Print and shaded views of the part. All mm, measured from the part's lowest x, y and z. A direction names the side the tool comes from. Round coordinates to 2 decimals unless told otherwise and drop trailing zeros. Order: outer loops, then holes, each group sorted by start corner. A loop starts at its lowest first (then second) coordinate and runs counter-clockwise, first axis right, second up. Notation, with made-up numbers: (85.5, 3.25) - (109.5, 3.25) arc R5 cw to (109.5, 10.25) - close; hole circle Ø2 at (-16, -25.75). An arc over 180 degrees is marked (long way). Return JSON: item names as keys, results as strings. Group by question number.
Item 1: Saw through at C-C on x = 10. List the corners of the cut face in (y, z).
Item 2: Saw through at B-B on z = 10.5. List the corners of the cut face in (x, y).
Item 3: Saw through at D-D on z = 18.5. List the corners of the cut face in (x, y), and give its area (3 significant figures).
Item 4: Tool access for the marked faces 5, 6, 7 and 8: list every direction of +Z, -Z, +X, -X, +Y, -Y with a clear straight run to the whole face (end or side of a thin tool).
Item 5: Saw through at A-A on y = 8.5. List the corners of the cut face in (x, z).
Item 6: Drop flat-ended pins along their axis: pin 1 (25 mm diameter, centred on x = 53, z = 34.5, fed in from -Y); pin 2 (11.5 mm diameter, centred on x = 108, z = 60, fed in from +Y); pin 3 (1.5 mm diameter, centred on y = 11.5, z = 52.5, fed in from +X). Give the stop position or say it passes through.
Item 7: Probe probe 1 along Y at (x, z) = (46, 16); probe 2 along Z at (x, y) = (112, 8) (1 decimal); probe 3 along Y at (x, z) = (103, 28.5). List the from-to ranges inside material, lowest first.
Item 8: Two-plate mould, pull along Z, no slides. Class the marked faces 1, 2, 3 and 4: released by +Z, released by -Z, zero draft, split by the parting line, or undercut.
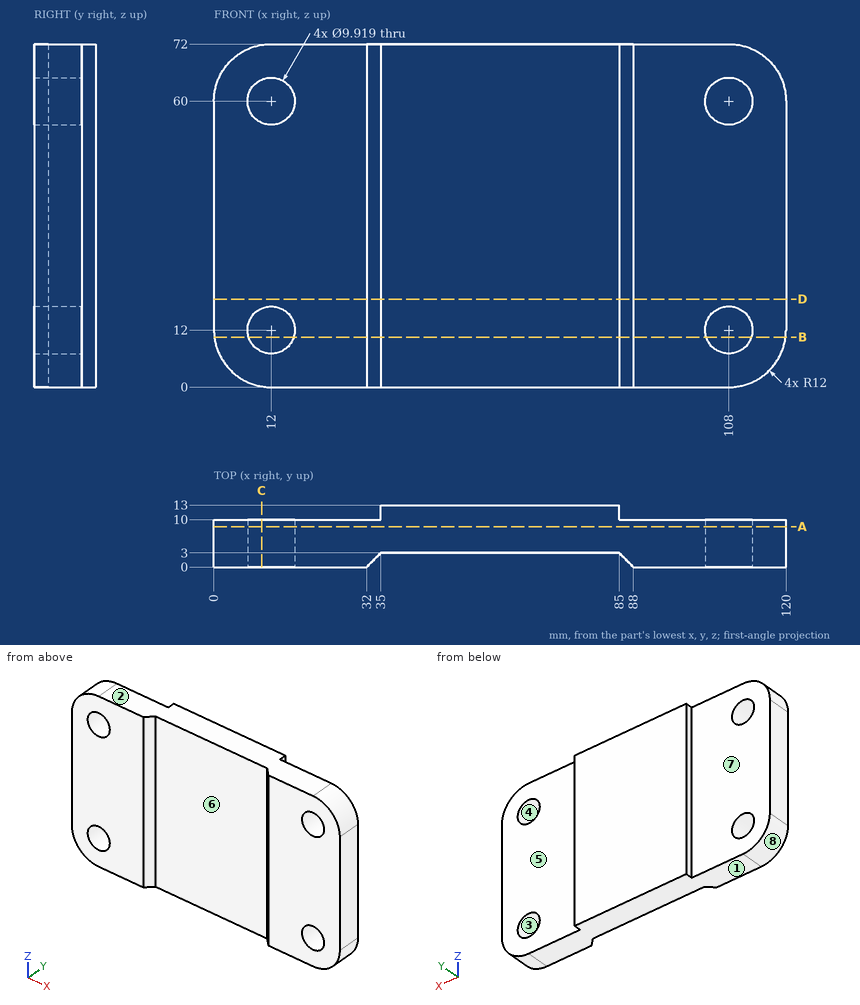
Filled in:
{
 "1": {"outline": "(0, 0.17) - (10, 0.17) - (10, 7.46) - (0, 7.46) - close; (0, 16.54) - (10, 16.54) - (10, 55.46) - (0, 55.46) - close; (0, 64.54) - (10, 64.54) - (10, 71.83) - (0, 71.83) - close"},
 "2": {"outline": "(0.09, 0) - (7.27, 0) - (7.27, 10) - (0.09, 10) - close; (16.73, 0) - (32, 0) - (35, 3) - (85, 3) - (88, 0) - (103.27, 0) - (103.27, 10) - (85, 10) - (85, 13) - (35, 13) - (35, 10) - (16.73, 10) - close; (112.73, 0) - (119.91, 0) - (119.91, 10) - (112.73, 10) - close"},
 "3": {"outline": "(0, 0) - (32, 0) - (35, 3) - (85, 3) - (88, 0) - (120, 0) - (120, 10) - (85, 10) - (85, 13) - (35, 13) - (35, 10) - (0, 10) - close", "area": "1,190 mm^2"},
 "4": {"face 5": "+Z, -Z, +X, +Y", "face 6": "+Z, -Z, -Y", "face 7": "+Z, -Z, -X, +Y", "face 8": "-Z, -X, +Y, -Y"},
 "5": {"outline": "(0, 12) arc R12 ccw to (12, 0) - (108, 0) arc R12 ccw to (120, 12) - (120, 60) arc R12 ccw to (108, 72) - (12, 72) arc R12 ccw to (0, 60) - close; hole circle Ø9.92 at (12, 12); hole circle Ø9.92 at (12, 60); hole circle Ø9.92 at (108, 12); hole circle Ø9.92 at (108, 60)"},
 "6": {"pin 1": "stops at y = 3", "pin 2": "stops at y = 10", "pin 3": "stops at x = 85"},
 "7": {"probe 1": "y = 3 to 13", "probe 2": "z = 0.7 to 9.1, 14.9 to 57.1, 62.9 to 71.3", "probe 3": "y = 0 to 10"},
 "8": {"face 1": "released by -Z", "face 2": "released by +Z", "face 3": "undercut", "face 4": "undercut"}
}
